from build123d import *

# Parameters (mm, degrees)
SKETCH1_R           = 5.5
BOSS_EXTRUDE1_DEPTH = 1
SKETCH2_R           = 8
BOSS_EXTRUDE2_DEPTH = 16
SKETCH3_W           = 8.2
SKETCH3_H           = 8.2
CUT_EXTRUDE1_DEPTH  = 21.420577857
SKETCH4_R           = 2
CUT_EXTRUDE2_DEPTH  = 25


with BuildPart() as part:
    # Sketch1 → Boss-Extrude1 (new body)
    with BuildSketch(Plane(origin=(0, 0, 0), x_dir=(1, 0, 0), z_dir=(0, 1, 0))):
        with Locations(Location((0, 0, 0), (0, 0, 270))):
            Circle(SKETCH1_R)
    extrude(amount=BOSS_EXTRUDE1_DEPTH)

    # Sketch2 → Boss-Extrude2 (add)
    with BuildSketch(Plane(origin=(0, 0, 0), x_dir=(-1, 0, 0), z_dir=(0, -1, 0))):
        with Locations(Location((0, 0, 0), (0, 0, 90))):
            Circle(SKETCH2_R)
    extrude(amount=BOSS_EXTRUDE2_DEPTH)

    # Sketch3 → Cut-Extrude1 (cut, through all)
    with BuildSketch(Plane.XZ.offset(16)):
        Rectangle(SKETCH3_W, SKETCH3_H)
    extrude(amount=-CUT_EXTRUDE1_DEPTH, mode=Mode.SUBTRACT)

    # Sketch4 → Cut-Extrude2 (cut, through all)
    with BuildSketch(Plane.ZY.offset(8)):
        with Locations(Location((0, -12, 0), (0, 0, 90))):
            Circle(SKETCH4_R)
    extrude(amount=-CUT_EXTRUDE2_DEPTH, mode=Mode.SUBTRACT)


solid = part.part
Part model, mm, in its own coordinate system. A direction names the side the tool comes from. Give positions to 0.01 mm unless a question says otherwise; leave off trailing zeros. Loops run counter-clockwise (first coordinate to the right, second up) from the corner with the lowest first, then second, coordinate; pieces in that order, holes last. Notation, with made-up numbers: (15.25, -28) -> (64.25, -28) arc R25 ccw to (64.25, 10) -> close; hole circle Ø3 at (-6, 47.25). An arc over 180 degrees is marked (long way). Write each question's results on one line, items separated by ' | '. Start each with the question number.
Q1. Band-saw the part on C-C on y = -12. List the corners of the cut face in (x, z).
Q2. Band-saw the part on A-A on x = 0. List the corners of the cut face in (y, z), plus the area to 3 significant figures.
Q3. Wall check: L1, parallel to Z at x = -0.25, y = -9; L2, parallel to X at y = -3.25, z = -3.5. Give the ranges that are in metal, low to high.
Q4. Band-saw the part on B-B on z = 0. List the corners of the cut face in (x, y).
Q5. Pin check, flat tips, straight feed: P1, Ø6, axis at x = 2.5, z = 1.5, coming from the +Y side; P2, Ø2.5, axis at y = -6.5, z = 1.5, coming from the +X side; P3, Ø6, axis at x = -4.5, y = -10, coming from the +Z side; P4, Ø2.5, axis at x = -1.5, y = -10.5, coming from the +Z side. Stop position of each tip, or through.
Q6. Band-saw the part on D-D on y = -5. List the corners of the cut face in (x, z), plus the area to 3 significant figures.
Q7. Pull direction Y, two halves, no side cores. Call faces 4 (the face through (-6, -12, -2)), 5 (the face through (6.026, -10.153, 0.766)), 6 (the face through (0, -8, 4.1)), 7 (the face through (-5, 1, 0)): +Y half, -Y half, draft (parallel to the pull), parting line (faces both ways), or undercut.
Q8. Which spindle directions (+Z, -Z, +X, -X, +Y, -Y) get a long thin tool onto all of the face, cutting with end or side? Do faces 1 (the face through (4.1, -8, 0)), 2 (the face through (5.5, 0.5, 0.1)), 3 (the face through (-0.1, 0.5, 5.5)). Say none if no direction does.
Results are:
1) outline: (-7.75, -2) arc R8 ccw to (7.75, -2) -> (4.1, -2) -> (4.1, -4.1) -> (-4.1, -4.1) -> (-4.1, -2) -> close; (-7.75, 2) -> (-4.1, 2) -> (-4.1, 4.1) -> (4.1, 4.1) -> (4.1, 2) -> (7.75, 2) arc R8 ccw to start
2) outline: (-16, -8) -> (0, -8) -> (0, -5.5) -> (1, -5.5) -> (1, -4.1) -> (-16, -4.1) -> close; (-16, 4.1) -> (1, 4.1) -> (1, 5.5) -> (0, 5.5) -> (0, 8) -> (-16, 8) -> close | area: 128 mm²
3) L1: z = -8 to -4.1, 4.1 to 8 | L2: x = -7.19 to -4.1, 4.1 to 7.19
4) outline: (-8, -16) -> (-4.1, -16) -> (-4.1, -14) -> (-8, -14) -> close; (-8, -10) -> (-4.1, -10) -> (-4.1, 1) -> (-5.5, 1) -> (-5.5, 0) -> (-8, 0) -> close; (4.1, -16) -> (8, -16) -> (8, -14) -> (4.1, -14) -> close; (4.1, -10) -> (8, -10) -> (8, 0) -> (5.5, 0) -> (5.5, 1) -> (4.1, 1) -> close
5) P1: stops at y = 1 | P2: stops at x = 8 | P3: stops at z = 7.86 | P4: stops at z = 8
6) outline: circle Ø16 at (0, 0); hole (-4.1, -4.1) -> (4.1, -4.1) -> (4.1, 4.1) -> (-4.1, 4.1) -> close | area: 134 mm²
7) face 4: undercut | face 5: undercut | face 6: draft | face 7: +Y half
8) face 1: +Y, -Y | face 2: +X, +Y | face 3: +Z, +Y
